CAD build for the part. Positions are in the model's coordinates, mm. Face numbers are marked on the shaded views. A direction names the side the tool comes from. Give positions to 0.01 mm unless a question says otherwise; leave off trailing zeros. Order: outer loops, then holes, each group sorted by start corner. A loop starts at its lowest first (then second) coordinate and runs counter-clockwise, first axis right, second up. Notation, with made-up numbers: (-3.75, 41) -> (25.25, 41) arc R10 cw to (25.25, 45) -> close; hole circle Ø1 at (18.5, 77.25). An arc over 180 degrees is marked (long way). Use one line per item in the form item = value. Start each with the question number.
1) Cut at A-A, the plane x = 0. Give the cut face in (y, z).
2) Cut at C-C, the plane y = 180. Give the cut face in (x, z), and give its area (3 significant figures).
3) Cut at D-D, the plane x = -12.5. Give the cut face in (y, z), and give its area (3 significant figures).
4) Mould opens along X. For the marked faces 1, 2, 3 and 4 say: pulls with the +X half, pulls with the -X half, needs draft (parallel to the pull), parting line crosses it, or undercut.
5) Cut at B-B, the plane y = 18. Give the cut face in (x, z), and give its area (3 significant figures).
6) Drop flat-ended pins along their axis: P1, Ø4, axis at x = -12.5, y = 65.5, coming from the -Z side; P2, Ø9, axis at y = 75.5, z = -20.5, coming from the +X side; P3, Ø2, axis at x = 25.5, y = 105.5, coming from the -Z side; P4, Ø6, axis at x = 0, y = 180, coming from the +Z side. Give the stop position or say it passes through.
7) Tool access for the marked faces 5, 6, 7, 8 and 9: list every direction of +Z, -Z, +X, -X, +Y, -Y with a clear straight run to the whole face (end or side of a thin tool).
8) Probe line 1 (Y direction, x = 0, z = 8.25); line 2 (Z direction, x = 20, y = 90.5); line 3 (Y direction, x = -6.5, z = -24). List the from-to ranges inside material, lowest first.
from build123d import *

# Parameters (mm, degrees)
SKETCH1_R           = 5
BOSS_EXTRUDE1_DEPTH = 15
SKETCH2_W           = 80
SKETCH2_H           = 10
BOSS_EXTRUDE2_DEPTH = 118
SKETCH3_W           = 20
SKETCH3_H           = 30
SKETCH3_W_2         = 5
SKETCH3_H_2         = 50
BOSS_EXTRUDE3_DEPTH = 30


with BuildPart() as part:
    # Sketch1 → Boss-Extrude1 (new body)
    with BuildSketch(Plane.XY):
        with BuildLine():
            Line((-40, 10), (-40, 0))
            Line((-40, 0), (40, 0))
            Line((40, 0), (40, 10))
            Line((40, 10), (35, 10))
            Line((35, 10), (35, 90))
            Line((35, 90), (9.656157585, 182.599734734))
            ThreePointArc((9.656157585, 182.599734734), (0.020772469, 189.999978425), (-9.645273695, 182.639828659))
            Line((-9.645273695, 182.639828659), (-35, 90))
            Line((-35, 90), (-35, 10))
            Line((-35, 10), (-40, 10))
        make_face()
        with Locations((0, 180)):
            Circle(SKETCH1_R, mode=Mode.SUBTRACT)
    extrude(amount=BOSS_EXTRUDE1_DEPTH)

    # Sketch2 → Boss-Extrude2 (add)
    with BuildSketch(Plane(origin=(0, 0, 0), x_dir=(-1, 0, 0), z_dir=(0, 0, -1))):
        with Locations((0, 5)):
            Rectangle(SKETCH2_W, SKETCH2_H)
    extrude(amount=BOSS_EXTRUDE2_DEPTH)

    # Sketch3 → Boss-Extrude3 (add)
    with BuildSketch(Plane(origin=(0, 0, 0), x_dir=(-1, 0, 0), z_dir=(0, 0, -1))):
        with Locations((0, 25)):
            Rectangle(SKETCH3_W, SKETCH3_H)
        with Locations((-12.5, 75)):
            Rectangle(SKETCH3_W_2, SKETCH3_H_2)
        with Locations((12.5, 75)):
            Rectangle(SKETCH3_W_2, SKETCH3_H_2)
    extrude(amount=BOSS_EXTRUDE3_DEPTH)


solid = part.part
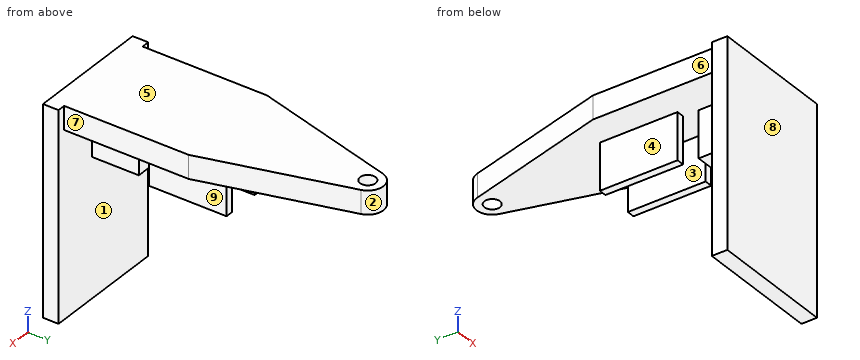
Result:
q1.outline = (0, -118) -> (10, -118) -> (10, -30) -> (40, -30) -> (40, 0) -> (175, 0) -> (175, 15) -> (0, 15) -> close; (185, 0) -> (190, 0) -> (190, 15) -> (185, 15) -> close
q2.outline = (-10.37, 0) -> (-5, 0) -> (-5, 15) -> (-10.37, 15) -> close; (5, 0) -> (10.37, 0) -> (10.37, 15) -> (5, 15) -> close
q2.area = 161 mm²
q3.outline = (0, -118) -> (10, -118) -> (10, 0) -> (50, 0) -> (50, -30) -> (100, -30) -> (100, 0) -> (172.21, 0) -> (172.21, 15) -> (0, 15) -> close
q3.area = 5,260 mm²
q4.face_1 = needs draft
q4.face_2 = parting line crosses it
q4.face_3 = undercut
q4.face_4 = pulls with the -X half
q5.outline = (-35, 0) -> (-10, 0) -> (-10, -30) -> (10, -30) -> (10, 0) -> (35, 0) -> (35, 15) -> (-35, 15) -> close
q5.area = 1,650 mm²
q6.P1 = -30
q6.P2 = 15
q6.P3 = 0
q6.P4 = through
q7.face_5 = +Z, +X, -X, +Y, -Y
q7.face_6 = +Z, -Z, -X, +Y
q7.face_7 = +Z, -Z, +X, +Y
q7.face_8 = +Z, -Z, +X, -X, -Y
q7.face_9 = -Z, +X, +Y
q8.line_1 = 0 to 175, 185 to 190
q8.line_2 = 0 to 15
q8.line_3 = 0 to 40
